The listing builds one solid part. Answer for the finished solid, in the listing's coordinates (mm). Face numbers are marked on the shaded views. A direction names the side the tool comes from. Give positions to 0.01 mm unless a question says otherwise; leave off trailing zeros. Write each loop counter-clockwise with the first axis right and the second up, starting at its lowest first coordinate (ties: lowest second). Pieces come first, ordered by that corner, then holes. Notation, with made-up numbers: (-1, 34.5) -> (51, 34.5) arc R21 ccw to (51, 69.5) -> close; hole circle Ø7 at (-13, 12). An arc over 180 degrees is marked (long way). One line per question, with ' | ' between items.
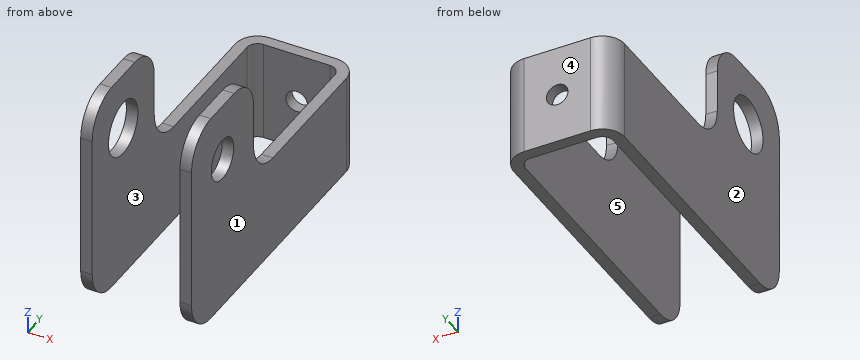
from build123d import *

# Parameters (mm, degrees)
SKETCH1_W                    = 7.7
SKETCH1_H                    = 7
BASE_FLANGE1_DEPTH           = 0.8
EDGE_FLANGE2_STRIP_W         = 4.6732
EDGE_FLANGE2_STRIP_H         = 0.8
EDGE_FLANGE2_STRIP_CUT_DEPTH = 7
EDGE_FLANGE2_DEPTH           = 7
EDGE_FLANGE2_FLAT_DEPTH      = 0.8
HOLE1_START                  = -1.85
HOLE1_OUTLINE_R              = 1.45
HOLE1_DEPTH                  = 0.8
HOLE4_START                  = -0.8
HOLE4_OUTLINE_R              = 0.75
HOLE4_DEPTH                  = 0.8
FILLET1_R                    = 2.5
SKETCH24_R                   = 1.9
CUT_EXTRUDE1_DEPTH           = 1


# Read off the part's stored shape, not the designer's step: Hole1, Hole4
# Sheet-metal steps are written as plain solids
with BuildPart() as part:
    # Sketch1 → Base-Flange1 (new body)
    with BuildSketch(Plane(origin=(0, 0, 0), x_dir=(1, 0, 0), z_dir=(0, 1, 0))):
        with Locations((2, -0.01953125)):
            Rectangle(SKETCH1_W, SKETCH1_H)
    extrude(amount=-BASE_FLANGE1_DEPTH)

    # Edge-Flange2 strip (across the edge) → Edge-Flange2 strip cut (cut)
    with BuildSketch(Plane(origin=(-1.85, -0.8, 3.51953125), x_dir=(1, 0, 0), z_dir=(0, 0, -1))):
        with Locations((-0.8, -0.4)):
            Rectangle(EDGE_FLANGE2_STRIP_W, EDGE_FLANGE2_STRIP_H)
    edge_flange2_strip_cut = extrude(amount=EDGE_FLANGE2_STRIP_CUT_DEPTH, mode=Mode.SUBTRACT)

    # Edge-Flange2 bend section (across the edge) → Edge-Flange2 (add)
    with BuildSketch(Plane(origin=(-1.85, -0.8, 3.51953125), x_dir=(1, 0, 0), z_dir=(0, 0, -1))):
        with BuildLine():
            Line((0, 0.7366), (0.8, 0.7366))
            ThreePointArc((0.8, 0.7366), (1.015745145, 0.215745145), (1.5366, 0))
            Line((1.5366, 0), (1.5366, -0.8))
            ThreePointArc((1.5366, -0.8), (0.45005972, -0.34994028), (0, 0.7366))
        make_face()
    edge_flange2 = extrude(amount=EDGE_FLANGE2_DEPTH)

    # Edge-Flange2 profile (on flange) → Edge-Flange2 flat (add)
    with BuildSketch(Plane(origin=(-1.85, -0.8, 0), x_dir=(0, 0, -1), z_dir=(-1, 0, 0))):
        with BuildLine():
            Line((3.48046875, 0.7366), (3.48046875, 20.7))
            Line((3.48046875, 20.7), (-3.51953125, 20.7))
            Line((-3.51953125, 20.7), (-11.51953125, 20.7))
            Line((-11.51953125, 20.7), (-11.51953125, 12.7))
            Line((-11.51953125, 12.7), (-6.01953125, 12.7))
            ThreePointArc((-6.01953125, 12.7), (-4.251764297, 11.967766953), (-3.51953125, 10.2))
            Line((-3.51953125, 10.2), (-3.51953125, 0.7366))
            Line((-3.51953125, 0.7366), (3.48046875, 0.7366))
        make_face()
    edge_flange2_flat = extrude(amount=-EDGE_FLANGE2_FLAT_DEPTH)

    # Hole1 outline → Hole1 (cut)
    with BuildSketch(Plane.YZ.offset(HOLE1_START)):
        with Locations((-17.5, 7.51953125)):
            Circle(HOLE1_OUTLINE_R)
    hole1 = extrude(amount=HOLE1_DEPTH, mode=Mode.SUBTRACT)

    # Hole4 outline → Hole4 (cut)
    with BuildSketch(Plane(origin=(0, 0, 0), x_dir=(1, 0, 0), z_dir=(0, 1, 0)).offset(HOLE4_START)):
        with Locations((2, -0.01953125)):
            Circle(HOLE4_OUTLINE_R)
    extrude(amount=HOLE4_DEPTH, mode=Mode.SUBTRACT)

    # Mirror1: Edge-Flange2 strip cut, Edge-Flange2, Edge-Flange2 flat, Hole1 across plane
    add(edge_flange2_strip_cut.mirror(Plane(origin=(2, 0, 0), x_dir=(0, 0, 1), z_dir=(1, 0, 0))), mode=Mode.SUBTRACT)
    add(edge_flange2.mirror(Plane(origin=(2, 0, 0), x_dir=(0, 0, 1), z_dir=(1, 0, 0))))
    add(edge_flange2_flat.mirror(Plane(origin=(2, 0, 0), x_dir=(0, 0, 1), z_dir=(1, 0, 0))))
    add(hole1.mirror(Plane(origin=(2, 0, 0), x_dir=(0, 0, 1), z_dir=(1, 0, 0))), mode=Mode.SUBTRACT)

    # Fillet1
    fillet1_edges = [part.edges().sort_by_distance(p)[0] for p in [
        (-1.45, -21.5, -3.48046875),
        (-1.45, -21.5, 11.51953125),
        (-1.45, -13.5, 11.51953125),
        (5.45, -21.5, -3.48046875),
        (5.45, -13.5, 11.51953125),
        (5.45, -21.5, 11.51953125),
    ]]
    fillet(fillet1_edges, radius=FILLET1_R)

    # Sketch24 → Cut-Extrude1 (cut)
    with BuildSketch(Plane(origin=(-1.85, 0, 0), x_dir=(0, 0, -1), z_dir=(1, 0, 0))):
        with Locations(Location((-7.51953125, -17.5, 0), (0, 0, 270))):
            Circle(SKETCH24_R)
    extrude(amount=CUT_EXTRUDE1_DEPTH, mode=Mode.SUBTRACT)


solid = part.part
Item 1: Consider line 1 (Z direction, x = -1.6, y = -17.5); line 2 (X direction, y = -3.25, z = -1.25); line 3 (Z direction, x = 2, y = -0.45). Determine where each line is inside the solid, lowest interval first. Write a range as [from, to].
Answers below:
line 1: [-3.48, 5.62], [9.42, 11.52] | line 2: [-1.85, -1.05], [5.05, 5.85] | line 3: [-3.48, -0.73], [0.77, 3.52]
Item 2: Determine the mould class of the marked faces 1, 2 and 3 for opening direction X: pulls with the +X half, pulls with the -X half, needs draft (parallel to the pull), parting line crosses it, or undercut.
Answers below:
face 1: pulls with the +X half | face 2: pulls with the -X half | face 3: undercut
Item 3: Find section B-B (z = 9.75). Write down the section's boundary in (x, y), then the cut area to 3 significant figures.
Answers below:
outline: (-1.85, -21.39) -> (-1.05, -21.39) -> (-1.05, -13.61) -> (-1.85, -13.61) -> close; (5.05, -21.39) -> (5.85, -21.39) -> (5.85, -13.61) -> (5.05, -13.61) -> close | area: 12.5 mm²
Item 4: Flat-ended cylindrical pins translate along their axes: pin 1 (2 mm diameter, centred on x = 0, z = -1, fed in from +Y); pin 2 (2.5 mm diameter, centred on x = 1, z = 1.5, fed in from -Y); pin 3 (0.6 mm diameter, centred on x = 5.5, z = 7, fed in from +Y); pin 4 (1.2 mm diameter, centred on x = 2, z = 0.02, fed in from +Y). Find the tip coordinate at first contact, or state that the pin passes through.
Answers below:
pin 1: y = 0 | pin 2: y = -0.8 | pin 3: y = -13.5 | pin 4: through
Item 5: Find section A-A (y = -9.5). Write down the section's boundary in (x, z).
Answers below:
outline: (-1.85, -3.48) -> (-1.05, -3.48) -> (-1.05, 3.52) -> (-1.85, 3.52) -> close; (5.05, -3.48) -> (5.85, -3.48) -> (5.85, 3.52) -> (5.05, 3.52) -> close
Item 6: Find section C-C (z = 1.5). Write down the section's boundary in (x, y), then the cut area to 3 significant figures.
Answers below:
outline: (-1.85, -21.5) -> (-1.05, -21.5) -> (-1.05, -1.54) arc R0.74 cw to (-0.31, -0.8) -> (4.31, -0.8) arc R0.74 cw to (5.05, -1.54) -> (5.05, -21.5) -> (5.85, -21.5) -> (5.85, -1.54) arc R1.54 ccw to (4.31, 0) -> (-0.31, 0) arc R1.54 ccw to (-1.85, -1.54) -> close | area: 38.5 mm²
Item 7: A tool of negligible diameter and unlimited length cuts with its end or side. For the marked faces 4 and 5, from which of +Z, -Z, +X, -X, +Y, -Y can it reach the whole face along a straight path? Write none if from no direction.
Answers below:
face 4: +Z, -Z, +X, -X, +Y | face 5: +Z, -Z, -Y
Item 8: Find section D-D (y = -16.5). Write down the section's boundary in (x, z), then the cut area to 3 significant figures.
Answers below:
outline: (-1.85, -3.48) -> (-1.05, -3.48) -> (-1.05, 5.9) -> (-1.85, 5.9) -> close; (-1.85, 9.14) -> (-1.05, 9.14) -> (-1.05, 11.52) -> (-1.85, 11.52) -> close; (5.05, -3.48) -> (5.85, -3.48) -> (5.85, 6.47) -> (5.05, 6.47) -> close; (5.05, 8.57) -> (5.85, 8.57) -> (5.85, 11.52) -> (5.05, 11.52) -> close | area: 19.7 mm²
